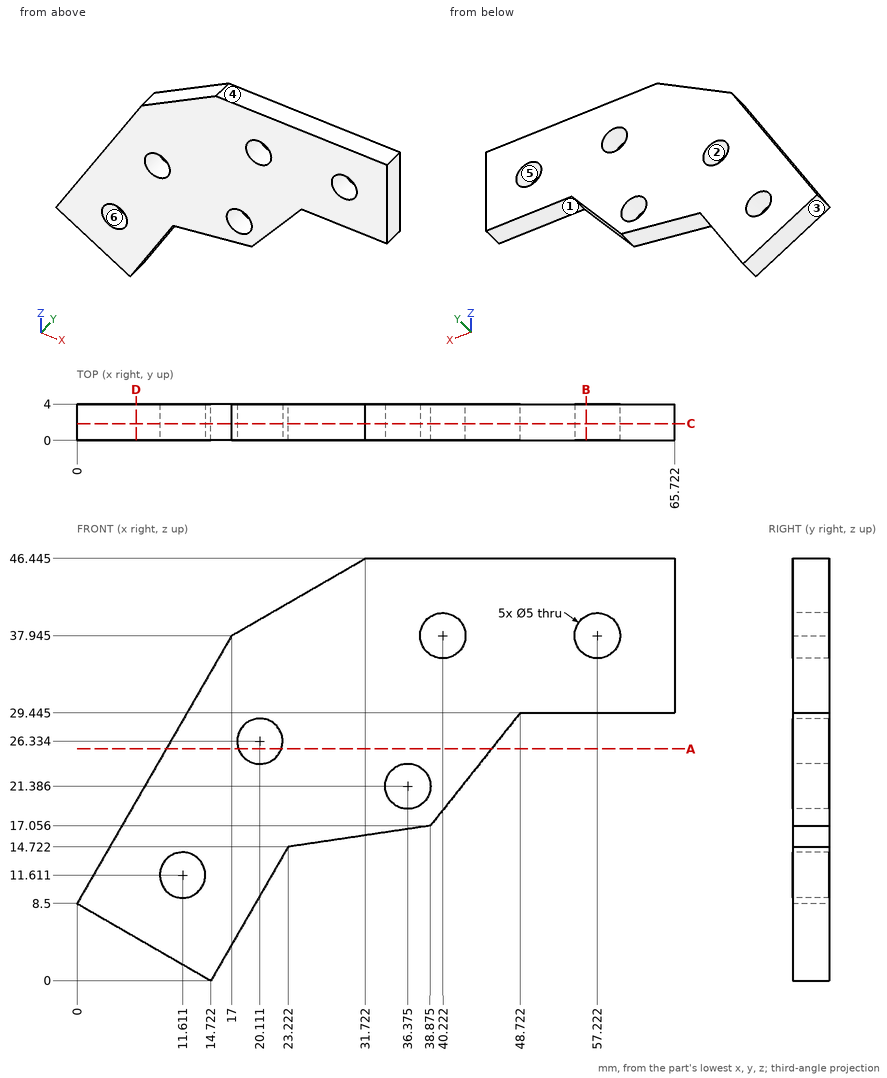
Study the drawing (mm; zero at the part's minimum x, y, z) and answer. A direction names the side the tool comes from. Give positions to 0.01 mm unless a question says otherwise; leave off trailing zeros. Loops run counter-clockwise (first coordinate to the right, second up) from the corner with the lowest first, then second, coordinate; pieces in that order, holes last. Notation, with made-up numbers: (-35, -34) - (-24, -34) arc R19 cw to (-24, -8) - close; hole circle Ø1 at (42.25, -25). An arc over 180 degrees is marked (long way). Return JSON: item names as keys, results as strings. Group by question number.
1. Find section C-C (y = 1.85). Write down the section's boundary in (x, z) (1 decimal).
2. Find section D-D (x = 6.5). Write down the section's boundary in (y, z).
3. Given pin 1 Ø1.5 at (x, z) = (16.5, 13) entering from -Y; pin 2 Ø2 at (x, y) = (56.5, 1) entering from -Z (1 decimal), each flat-ended and moving along its own axis, determine where each tip first touches the part or whether it passes through.
4. Determine the mould class of the marked faces 3, 4, 5 and 6 for opening direction X: pulls with the +X half, pulls with the -X half, needs draft (parallel to the pull), parting line crosses it, or undercut.
5. Straight lines are drawn through the part: line 1 (Z direction, x = 57, y = 3.4) (1 decimal); line 2 (Z direction, x = 49.5, y = 3.2) (1 decimal); line 3 (Z direction, x = 56.5, y = 0.75) (1 decimal). For each, find the intervals that lie inside material, in ascending order. Write a range as [from, to].
6. Find section A-A (z = 25.5). Write down the section's boundary in (x, y) (1 decimal).
7. Which of the six approach directions +Z, -Z, +X, -X, +Y, -Y give full straight-line access (tool end or side, diameter ignored) to the marked faces 1 and 2?
8. Find section B-B (x = 56). Write down the section's boundary in (y, z) (1 decimal).
Verdict:
{
 "1": {"outline": "(0, 8.5) - (14.7, 0) - (23.2, 14.7) - (38.9, 17.1) - (48.7, 29.4) - (65.7, 29.4) - (65.7, 46.4) - (31.7, 46.4) - (17, 37.9) - close; hole circle Ø5 at (11.6, 11.6); hole circle Ø5 at (20.1, 26.3); hole circle Ø5 at (36.4, 21.4); hole circle Ø5 at (40.2, 37.9); hole circle Ø5 at (57.2, 37.9)"},
 "2": {"outline": "(0, 4.75) - (4, 4.75) - (4, 19.76) - (0, 19.76) - close"},
 "3": {"pin 1": "stops at y = 0", "pin 2": "stops at z = 29.4"},
 "4": {"face 3": "pulls with the -X half", "face 4": "needs draft", "face 5": "undercut", "face 6": "undercut"},
 "5": {"line 1": "z = [29.4, 35.5], [40.4, 46.4]", "line 2": "z = [29.4, 46.4]", "line 3": "z = [29.4, 35.6], [40.3, 46.4]"},
 "6": {"outline": "(9.8, 0) - (17.8, 0) - (17.8, 4) - (9.8, 4) - close; (22.5, 0) - (45.6, 0) - (45.6, 4) - (22.5, 4) - close"},
 "7": {"face 1": "-Z, +X, +Y, -Y", "face 2": "+Y, -Y"},
 "8": {"outline": "(0, 29.4) - (4, 29.4) - (4, 35.8) - (0, 35.8) - close; (0, 40.1) - (4, 40.1) - (4, 46.4) - (0, 46.4) - close"}
}
